For this review, take the finished solid that the model builds, in its own axes (mm). A direction names the side the tool comes from. Give positions to 0.01 mm unless a question says otherwise; leave off trailing zeros. Loops run counter-clockwise (first coordinate to the right, second up) from the corner with the lowest first, then second, coordinate; pieces in that order, holes last. Notation, with made-up numbers: (-5, 32.5) - (40, 32.5) arc R19 ccw to (40, 60.5) - close; hole circle Ø10 at (49.25, 79.25). An arc over 180 degrees is marked (long way). Use CSV: the item, a comma, the result in double quotes. Start each with the question number.
1. Wall thickness on line 1 (Z direction, x = 12, y = 10.75): over which ranges is the line inside the solid? List them lowest first.
2. Take a section at A-A on y = 9.5. Give the boundary of the cut face in (x, z), plus the area to 3 significant figures.
3. For pin 1 (2.5 mm diameter, centred on x = 17.5, y = 10, fed in from -Z), flat-tipped, find the tip position at first contact; note if it passes through.
4. For faces 4 (the cylindrical face through (34, 9.4, 0.5)), 5 (the flat face through (37.997, 9, 5)), list the 3-axis set-ups (+Z, -Z, +X, -X, +Y, -Y) from which the entire face can be reached by the end or side of a thin tool; tool diameter is ignored.
5. Mouldability with a two-part tool opening along Y and no side actions: class faces 1 (the flat face through (19, 10, 1)), 2 (the flat face through (19, 19, 5)), 3 (the flat face through (19, 10, 10)) as pulls with the +Y half, pulls with the -Y half, needs draft (parallel to the pull), parting line crosses it, or undercut.
6. Take a section at B-B on x = 28.5. Give the boundary of the cut face in (y, z), plus the area to 3 significant figures.
```python
from build123d import *

# Parameters (mm, degrees)
SKETCH_1_W          = 38
SKETCH_1_H          = 19
EXTRUDE_1_DEPTH     = 10
SKETCH_2_W          = 1.5
SKETCH_2_H          = 9
EXTRUDE_2_DEPTH     = 9
SKETCH_3_R          = 1.5
CUT_EXTRUDE_1_DEPTH = 52.322509681
FILLET_2_R          = 0.5
CUT_EXTRUDE_2_DEPTH = 1
SKETCH_5_W          = 59.581818612
SKETCH_5_H          = 24.32156281
SKETCH_5_W_2        = 37.996651515
SKETCH_5_H_2        = 19
CUT_EXTRUDE_3_DEPTH = 52.672042731


with BuildPart() as part:
    # 草图1 → 凸台-拉伸1 (new body)
    with BuildSketch(Plane.XY):
        with Locations((19, 9.5)):
            Rectangle(SKETCH_1_W, SKETCH_1_H)
    extrude(amount=EXTRUDE_1_DEPTH)

    # 草图2 → 凸台-拉伸2 (add)
    with BuildSketch(Plane(origin=(38, 0, 0), x_dir=(0, 0, -1), z_dir=(1, 0, 0))):
        with Locations((-2.75, 9.5)):
            Rectangle(SKETCH_2_W, SKETCH_2_H)
    extrude_2 = extrude(amount=EXTRUDE_2_DEPTH)

    # 草图3 → 切除-拉伸1 (cut, through all)
    with BuildSketch(Plane(origin=(0, 0, 2), x_dir=(-1, 0, 0), z_dir=(0, 0, -1))):
        with Locations((-42.5, 9.5)):
            Circle(SKETCH_3_R)
    cut_extrude_1 = extrude(amount=-CUT_EXTRUDE_1_DEPTH, mode=Mode.SUBTRACT)

    # 镜向3: 凸台-拉伸2, 切除-拉伸1 across plane
    add(extrude_2.mirror(Plane(origin=(19, 0, 0), x_dir=(0, 0, 1), z_dir=(1, 0, 0))))
    add(cut_extrude_1.mirror(Plane(origin=(19, 0, 0), x_dir=(0, 0, 1), z_dir=(1, 0, 0))), mode=Mode.SUBTRACT)

    # 圆角2
    fillet_2_edges = [part.edges().sort_by_distance(p)[0] for p in [
        (38, 5, 2.75),
        (38, 14, 2.75),
        (47, 5, 2.75),
        (47, 14, 2.75),
        (-9, 14, 2.75),
        (-9, 5, 2.75),
        (0, 5, 2.75),
        (0, 14, 2.75),
        (0, 19, 5),
        (38, 19, 5),
        (38, 0, 5),
        (0, 0, 5),
    ]]
    fillet(fillet_2_edges, radius=FILLET_2_R)

    # 草图4 → 切除-拉伸2 (cut)
    with BuildSketch(Plane(origin=(0, 0, 0), x_dir=(-1, 0, 0), z_dir=(0, 0, -1))):
        with BuildLine():
            Line((-30, 13.5), (-8, 13.5))
            ThreePointArc((-8, 13.5), (-4, 9.5), (-8, 5.5))
            Line((-8, 5.5), (-30, 5.5))
            ThreePointArc((-30, 5.5), (-34, 9.5), (-30, 13.5))
        make_face()
    extrude(amount=-CUT_EXTRUDE_2_DEPTH, mode=Mode.SUBTRACT)

    # 草图5 → 切除-拉伸3 (cut, through all)
    with BuildSketch(Plane(origin=(0, 0, 0), x_dir=(-1, 0, 0), z_dir=(0, 0, -1))):
        with Locations((-19.067430593, 9.084908835)):
            Rectangle(SKETCH_5_W, SKETCH_5_H)
        with Locations((-18.998325758, 9.5)):
            Rectangle(SKETCH_5_W_2, SKETCH_5_H_2, mode=Mode.SUBTRACT)
    extrude(amount=-CUT_EXTRUDE_3_DEPTH, mode=Mode.SUBTRACT)


solid = part.part
```
Check result:
1,line 1,"z = 1 to 10"
2,outline,"(0, 0) - (4, 0) - (4, 1) - (34, 1) - (34, 0) - (38, 0) - (38, 10) - (0, 10) - close"
2,area,"350 mm²"
3,pin 1,"stops at z = 1"
4,face 4,"-Z"
4,face 5,"+Z, -Z, +X, +Y, -Y"
5,face 1,"undercut"
5,face 2,"pulls with the +Y half"
5,face 3,"needs draft"
6,outline,"(0, 0) - (5.5, 0) - (5.5, 1) - (13.5, 1) - (13.5, 0) - (19, 0) - (19, 10) - (0, 10) - close"
6,area,"182 mm²"
